```python
from build123d import *

# Parameters (mm, degrees)
SALIENTE_EXTRUIR1_DEPTH = 10
CROQUIS3_R              = 4.1
CORTAR_EXTRUIR1_DEPTH   = 47.882832679
CROQUIS9_R              = 2.5
CORTAR_EXTRUIR6_DEPTH   = 47.882832679
SIMETR_A2_OUTLINE_R     = 4.1
SIMETR_A2_OUTLINE_R_2   = 2.5
SIMETR_A2_DEPTH         = 10
CROQUIS8_R              = 5
CORTAR_EXTRUIR2_DEPTH   = 10


# Read off the part's stored shape, not the designer's step: Simetría2
with BuildPart() as part:
    # Croquis2 → Saliente-Extruir1 (new body)
    with BuildSketch(Plane.XY):
        with BuildLine():
            Line((24, 0), (0, 0))
            Line((0, 0), (0, 14))
            ThreePointArc((0, 14), (13.564530661, 16.812621552), (24.892422825, 24.786716558))
            ThreePointArc((24.892422825, 24.786716558), (35.705553054, 24.055448723), (32.841827768, 13.602811951))
            ThreePointArc((32.841827768, 13.602811951), (26.404704634, 8.111941988), (24, 0))
        make_face()
    saliente_extruir1 = extrude(amount=SALIENTE_EXTRUIR1_DEPTH)

    # Croquis3 → Cortar-Extruir1 (cut, through all)
    with BuildSketch(Plane.XY):
        with Locations((30, 20)):
            Circle(CROQUIS3_R)
    cortar_extruir1 = extrude(amount=CORTAR_EXTRUIR1_DEPTH, mode=Mode.SUBTRACT)

    # Simetría1: Saliente-Extruir1, Cortar-Extruir1 across plane
    add(saliente_extruir1.mirror(Plane.ZX))
    add(cortar_extruir1.mirror(Plane.ZX), mode=Mode.SUBTRACT)

    # Croquis9 → Cortar-Extruir6 (cut, through all)
    with BuildSketch(Plane.XY):
        with Locations((18.25, 0)):
            Circle(CROQUIS9_R)
    extrude(amount=CORTAR_EXTRUIR6_DEPTH, mode=Mode.SUBTRACT)

    # Simetría2 outline → Simetría2 (add)
    with BuildSketch(Plane.XY):
        with BuildLine():
            Line((0, -14), (0, 14))
            ThreePointArc((0, 14), (-13.564530661, 16.812621552), (-24.892422825, 24.786716558))
            ThreePointArc((-24.892422825, 24.786716558), (-35.705553054, 24.055448723), (-32.841827768, 13.602811951))
            ThreePointArc((-32.841827768, 13.602811951), (-24, 0), (-32.841827768, -13.602811951))
            ThreePointArc((-32.841827768, -13.602811951), (-35.705553054, -24.055448723), (-24.892422825, -24.786716558))
            ThreePointArc((-24.892422825, -24.786716558), (-13.564530661, -16.812621552), (0, -14))
        make_face()
        with Locations((-30, -20)):
            Circle(SIMETR_A2_OUTLINE_R, mode=Mode.SUBTRACT)
        with Locations((-30, 20)):
            Circle(SIMETR_A2_OUTLINE_R, mode=Mode.SUBTRACT)
        with Locations((-18.25, 0)):
            Circle(SIMETR_A2_OUTLINE_R_2, mode=Mode.SUBTRACT)
    extrude(amount=SIMETR_A2_DEPTH)

    # Croquis8 → Cortar-Extruir2 (cut)
    with BuildSketch(Plane.XY):
        Circle(CROQUIS8_R)
    extrude(amount=CORTAR_EXTRUIR2_DEPTH, mode=Mode.SUBTRACT)


solid = part.part
```
Work out the finished part from the listing and answer in its coordinate system (mm). Round coordinates to 2 decimals unless told otherwise and drop trailing zeros. Order: outer loops, then holes, each group sorted by start corner. A loop starts at its lowest first (then second) coordinate and runs counter-clockwise, first axis right, second up.
Q1. A cutting plane is placed at A-A, the plane z = 1.75. Determine the outline of the cut face in (x, y).
Solution:
outline: (-32.84, -13.6) arc R7 ccw (long way) to (-24.89, -24.79) arc R34.12 cw to (24.89, -24.79) arc R7 ccw (long way) to (32.84, -13.6) arc R14.88 cw to (32.84, 13.6) arc R7 ccw (long way) to (24.89, 24.79) arc R34.12 cw to (-24.89, 24.79) arc R7 ccw (long way) to (-32.84, 13.6) arc R14.88 cw to start; hole circle Ø8.2 at (-30, -20); hole circle Ø8.2 at (-30, 20); hole circle Ø5 at (-18.25, 0); hole circle Ø10 at (0, 0); hole circle Ø5 at (18.25, 0); hole circle Ø8.2 at (30, -20); hole circle Ø8.2 at (30, 20)
Q2. Find the intervals of material crossed by line 1 along Y through (x, z) = (-30, 5.5); line 2 along Y through (x, z) = (0, 7.75); line 3 along X through (y, z) = (1.5, 1.5), in increasing order.
Solution:
line 1: y = -27 to -24.1, -15.9 to -11.94, 11.94 to 15.9, 24.1 to 27
line 2: y = -14 to -5, 5 to 14
line 3: x = -24.08 to -20.25, -16.25 to -4.77, 4.77 to 16.25, 20.25 to 24.08
Q3. A cutting plane is placed at B-B, the plane x = 18.25. Determine the outline of the cut face in (y, z).
Solution:
outline: (-19.29, 0) - (-2.5, 0) - (-2.5, 10) - (-19.29, 10) - close; (2.5, 0) - (19.29, 0) - (19.29, 10) - (2.5, 10) - close
Q4. A cutting plane is placed at C-C, the plane y = -4. Determine the outline of the cut face in (x, z).
Solution:
outline: (-24.55, 0) - (-3, 0) - (-3, 10) - (-24.55, 10) - close; (3, 0) - (24.55, 0) - (24.55, 10) - (3, 10) - close
Q5. A cutting plane is placed at D-D, the plane y = 20. Determine the outline of the cut face in (x, z), then the cut area to 3 significant figures.
Solution:
outline: (-37, 0) - (-34.1, 0) - (-34.1, 10) - (-37, 10) - close; (-25.9, 0) - (-19.32, 0) - (-19.32, 10) - (-25.9, 10) - close; (19.32, 0) - (25.9, 0) - (25.9, 10) - (19.32, 10) - close; (34.1, 0) - (37, 0) - (37, 10) - (34.1, 10) - close
area: 190 mm2
Q6. Given pin 1 Ø5 at (x, y) = (-7.5, 10) entering from -Z; pin 2 Ø1 at (x, z) = (22.5, 6) entering from +Y; pin 3 Ø2 at (x, z) = (-11.5, 3) entering from -Y; pin 4 Ø5 at (x, z) = (11, 8) entering from -Y, each flat-ended and moving along its own axis, determine where each tip first touches the part or whether it passes through.
Solution:
pin 1: stops at z = 0
pin 2: stops at y = 22.92
pin 3: stops at y = -16.37
pin 4: stops at y = -16.78
Q7. The mould has two halves that part along Y. Classify faces 1 (the flat face through (-1, -6, 0)), 2 (the cylindrical face through (35.6, -24.2, 4.9)): pulls with the +Y half, pulls with the -Y half, needs draft (parallel to the pull), parting line crosses it, or undercut.
Solution:
face 1: needs draft
face 2: undercut
